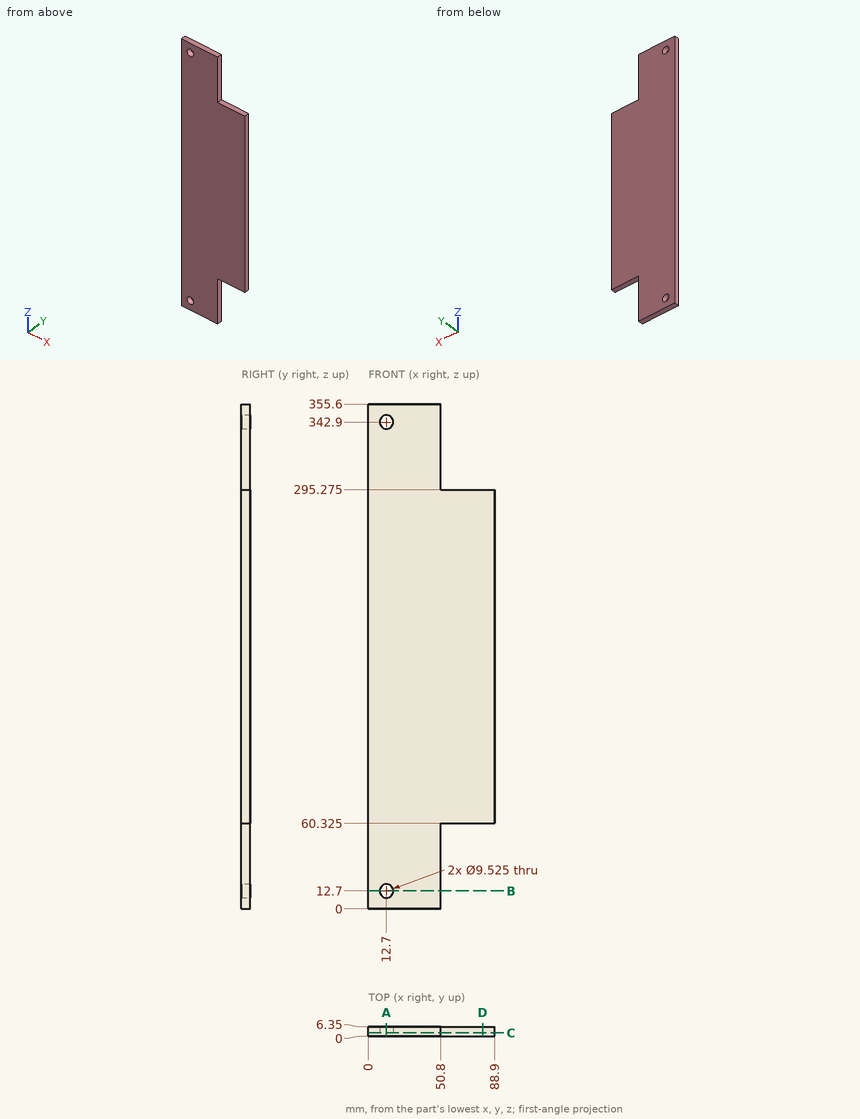
Print and shaded views of the part. All mm, measured from the part's lowest x, y and z. Coordinates: 2 decimals unless noted, no trailing zeros. Write each loop counter-clockwise with the first axis right and the second up, starting at its lowest first coordinate (ties: lowest second). Pieces come first, ordered by that corner, then holes. Notation, with made-up numbers: (6, 8.25) -> (50, 8.25) arc R31 cw to (50, 44.25) -> close; hole circle Ø10 at (-24, -17.5). An arc over 180 degrees is marked (long way). Use CSV: the item, a comma, the result in double quotes. Start each with the question number.
Q1. Drill centre lines: probe 1 along X at (y, z) = (3.75, 12.7); probe 2 along Z at (x, y) = (12, 1.25); probe 3 along Z at (x, y) = (11.5, 5.5). Where is each one in solid material? Low to high.
Q2. Cut at A-A, the plane x = 12.7. List the corners of the cut face in (y, z), then the cut area to 3 significant figures.
Q3. Flat gauge pins, fed straight in: pin 1 Ø3 at (y, z) = (2.5, 37.5) entering from +X; pin 2 Ø1 at (x, y) = (64, 5) entering from +Z (3 decimals); pin 3 Ø3 at (x, y) = (73, 3) entering from -Z (3 decimals). Where does each tip first touch, or does it go through?
Q4. Cut at C-C, the plane y = 2.25. List the corners of the cut face in (x, z) (1 decimal).
Q5. Cut at B-B, the plane z = 12.7. List the corners of the cut face in (x, y).
Q6. Cut at D-D, the plane x = 80.5. List the corners of the cut face in (y, z) (3 decimals), then the cut area to 3 significant figures.
Checked values:
1,probe 1,"x = 0 to 7.94, 17.46 to 50.8"
1,probe 2,"z = 0 to 7.99, 17.41 to 338.19, 347.61 to 355.6"
1,probe 3,"z = 0 to 8.09, 17.31 to 338.29, 347.51 to 355.6"
2,outline,"(0, 0) -> (6.35, 0) -> (6.35, 7.94) -> (0, 7.94) -> close; (0, 17.46) -> (6.35, 17.46) -> (6.35, 338.14) -> (0, 338.14) -> close; (0, 347.66) -> (6.35, 347.66) -> (6.35, 355.6) -> (0, 355.6) -> close"
2,area,"2,140 mm²"
3,pin 1,"stops at x = 50.8"
3,pin 2,"stops at z = 295.275"
3,pin 3,"stops at z = 60.325"
4,outline,"(0, 0) -> (50.8, 0) -> (50.8, 60.3) -> (88.9, 60.3) -> (88.9, 295.3) -> (50.8, 295.3) -> (50.8, 355.6) -> (0, 355.6) -> close; hole circle Ø9.5 at (12.7, 12.7); hole circle Ø9.5 at (12.7, 342.9)"
5,outline,"(0, 0) -> (7.94, 0) -> (7.94, 6.35) -> (0, 6.35) -> close; (17.46, 0) -> (50.8, 0) -> (50.8, 6.35) -> (17.46, 6.35) -> close"
6,outline,"(0, 60.325) -> (6.35, 60.325) -> (6.35, 295.275) -> (0, 295.275) -> close"
6,area,"1,490 mm²"
